```python
from build123d import *

# Parameters (mm, degrees)
BOSS_EXTRUDE1_DEPTH          = 4.7625
F_5_16_CLEARANCE_HOLE1_D     = 8.72998
F_5_16_CLEARANCE_HOLE2_D     = 8.72998
F_5_16_CLEARANCE_HOLE2_DEPTH = 50.8
F_5_16_CLEARANCE_HOLE2_TIP   = 2.622750593


with BuildPart() as part:
    # Sketch1 → Boss-Extrude1 (new body)
    with BuildSketch(Plane.XY):
        with BuildLine():
            Line((4.66554544, 6.421572393), (50.900866669, -27.170354776))
            ThreePointArc((50.900866669, -27.170354776), (52.656893621, -38.257472609), (41.569775788, -40.013499561))
            Line((41.569775788, -40.013499561), (-4.66554544, -6.421572393))
            ThreePointArc((-4.66554544, -6.421572393), (-6.421572393, 4.66554544), (4.66554544, 6.421572393))
        make_face()
    extrude(amount=BOSS_EXTRUDE1_DEPTH)

    # 5/16 Clearance Hole1 (through all)
    with Locations(Plane.XY.offset(4.7625)):
        with Locations((0, 0), (46.235321229, -33.591927169)):
            Hole(F_5_16_CLEARANCE_HOLE1_D / 2)

    # 5/16 Clearance Hole2
    with Locations(Plane(origin=(-478.115792966, -1361.199382297, 4.7625), x_dir=(0.9364927793764423, 0.3506868605690643, 0), z_dir=(0, 0, 1))):
        with Locations((956.625522808, 1059.411749502)):
            Hole(F_5_16_CLEARANCE_HOLE2_D / 2, depth=F_5_16_CLEARANCE_HOLE2_DEPTH)
            with Locations((0, 0, -(F_5_16_CLEARANCE_HOLE2_DEPTH + F_5_16_CLEARANCE_HOLE2_TIP / 2))):  # 118° drill point
                Cone(0, F_5_16_CLEARANCE_HOLE2_D / 2, F_5_16_CLEARANCE_HOLE2_TIP, mode=Mode.SUBTRACT)


solid = part.part
```
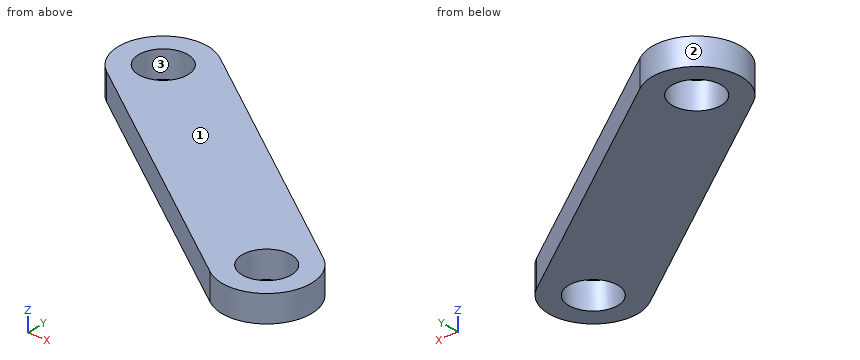
For this review, take the finished solid that the model builds, in its own axes (mm). Face numbers are marked on the shaded views. Round coordinates to 2 decimals unless told otherwise and drop trailing zeros. Write each loop counter-clockwise with the first axis right and the second up, starting at its lowest first coordinate (ties: lowest second). Pieces come first, ordered by that corner, then holes. Notation, with made-up numbers: (9, 38) -> (31, 38) arc R14 cw to (31, 60) -> close; hole circle Ø11 at (23.25, 89.25). An arc over 180 degrees is marked (long way). One line per question, with ' | ' between items. Start each with the question number.
1) Add section D-D (y = -16). Write out the cut boundary in (x, z).
2) Add section A-A (x = 0). Write out the cut boundary in (y, z).
3) Add section B-B (y = 0). Write out the cut boundary in (x, z) (1 decimal), and give its area (3 significant figures).
4) Wall thickness on line 1 along Y through (x, z) = (50, 0.7); line 2 along X through (y, z) = (-2.5, 1.8); line 3 along X through (y, z) = (-31, 3.95): over which ranges is each line inside the solid? List them lowest first.
5) Mouldability with a two-part tool opening along Y and no side actions: class the marked faces 1, 2 and 3 as +Y half, -Y half, draft (parallel to the pull), parting line (faces both ways), or undercut.
6) For pin 1 Ø1.5 at (y, z) = (-36.5, 2.5) entering from -X; pin 2 Ø1 at (x, z) = (3, 1.5) entering from -Y, all flat-tipped, find the tip position at first contact; note any pin that passes through.
7) Add section C-C (z = 1.4). Write out the cut boundary in (x, y) (1 decimal), and give its area (3 significant figures).
Reported:
1) outline: (8.52, 0) -> (35.53, 0) -> (35.53, 4.76) -> (8.52, 4.76) -> close
2) outline: (-9.81, 0) -> (-4.36, 0) -> (-4.36, 4.76) -> (-9.81, 4.76) -> close; (4.36, 0) -> (7.94, 0) -> (7.94, 4.76) -> (4.36, 4.76) -> close
3) outline: (-7.9, 0) -> (-4.4, 0) -> (-4.4, 4.8) -> (-7.9, 4.8) -> close; (4.4, 0) -> (13.5, 0) -> (13.5, 4.8) -> (4.4, 4.8) -> close | area: 60.5 mm²
4) line 1: y = -40.58 to -35.8, -31.38 to -26.52 | line 2: x = -7.53 to -3.58, 3.58 to 16.95 | line 3: x = 29.16 to 42.72, 49.75 to 53.74
5) face 1: draft | face 2: parting line | face 3: undercut
6) pin 1: stops at x = 35.7 | pin 2: stops at y = -12.35
7) outline: (-4.7, -6.4) -> (41.6, -40) arc R7.9 ccw to (50.9, -27.2) -> (4.7, 6.4) arc R7.9 ccw to start; hole circle Ø8.7 at (0, 0); hole circle Ø8.7 at (46.2, -33.6) | area: 985 mm²
